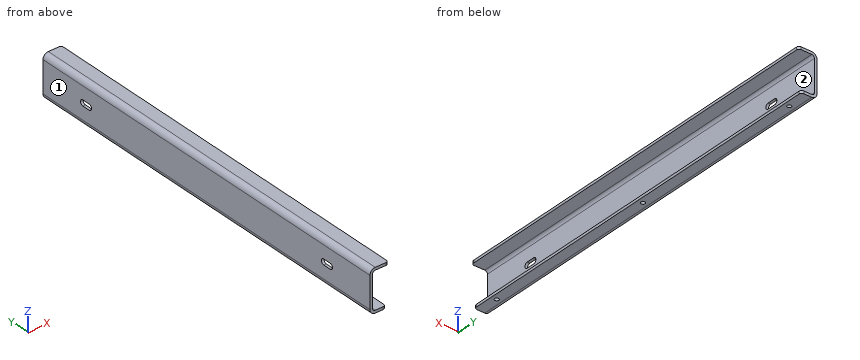
```python
from build123d import *

# Parameters (mm, degrees)
BASE_FLANGE1_DEPTH = 482.6
SKETCH6_R          = 2.45745
CUT_EXTRUDE1_DEPTH = 3.175
FILLET1_R          = 3.175
CUT_EXTRUDE3_DEPTH = 3.175


# Sheet-metal steps are written as plain solids
with BuildPart() as part:
    # Sketch1 → Base-Flange1 (new body)
    with BuildSketch(Plane(origin=(0, 0, 0), x_dir=(1, 0, 0), z_dir=(0, 1, 0))):
        with BuildLine():
            Line((0, 0), (-15.875, 0))
            ThreePointArc((-15.875, 0), (-20.365128061, 1.859871939), (-22.225, 6.35))
            Line((-22.225, 6.35), (-22.225, 44.45))
            ThreePointArc((-22.225, 44.45), (-20.365128061, 48.940128061), (-15.875, 50.8))
            Line((-15.875, 50.8), (-3.175, 50.8))
            Line((-3.175, 50.8), (-3.175, 47.625))
            Line((-3.175, 47.625), (-15.875, 47.625))
            ThreePointArc((-15.875, 47.625), (-18.12006403, 46.69506403), (-19.05, 44.45))
            Line((-19.05, 44.45), (-19.05, 6.35))
            ThreePointArc((-19.05, 6.35), (-18.12006403, 4.10493597), (-15.875, 3.175))
            Line((-15.875, 3.175), (0, 3.175))
            Line((0, 3.175), (0, 0))
        make_face()
    extrude(amount=BASE_FLANGE1_DEPTH)

    # Sketch6 → Cut-Extrude1 (cut)
    with BuildSketch(Plane(origin=(0, 0, -50.8), x_dir=(-1, 0, 0), z_dir=(0, 0, -1))):
        with Locations((9.525, 457.2)):
            Circle(SKETCH6_R)
        with Locations((9.525, 25.4)):
            Circle(SKETCH6_R)
        with Locations((9.525, 241.3)):
            Circle(SKETCH6_R)
    extrude(amount=-CUT_EXTRUDE1_DEPTH, mode=Mode.SUBTRACT)

    # Fillet1
    fillet1_edges = [part.edges().sort_by_distance(p)[0] for p in [
        (-3.175, 0, -49.2125),
        (0, 0, -1.5875),
        (-3.175, 482.6, -49.2125),
        (0, 482.6, -1.5875),
    ]]
    fillet(fillet1_edges, radius=FILLET1_R)

    # Sketch8 → Cut-Extrude3 (cut)
    with BuildSketch(Plane.ZY.offset(22.225)):
        with BuildLine():
            Line((-22.0265625, 423.8625), (-22.0265625, 414.3375))
            ThreePointArc((-22.0265625, 414.3375), (-25.4, 410.9640625), (-28.7734375, 414.3375))
            Line((-28.7734375, 414.3375), (-28.7734375, 423.8625))
            ThreePointArc((-28.7734375, 423.8625), (-25.4, 427.2359375), (-22.0265625, 423.8625))
        make_face()
        with BuildLine():
            Line((-28.7734375, 58.7375), (-28.7734375, 68.2625))
            ThreePointArc((-28.7734375, 68.2625), (-25.4, 71.6359375), (-22.0265625, 68.2625))
            Line((-22.0265625, 68.2625), (-22.0265625, 58.7375))
            ThreePointArc((-22.0265625, 58.7375), (-25.4, 55.3640625), (-28.7734375, 58.7375))
        make_face()
    extrude(amount=-CUT_EXTRUDE3_DEPTH, mode=Mode.SUBTRACT)


solid = part.part
```
Source: CAD feature listing. Evaluate the final solid. Frame: model axes, mm. Face numbers are marked on the shaded views. Coordinates: 2 decimals unless noted, no trailing zeros. Loops run counter-clockwise (first coordinate to the right, second up) from the corner with the lowest first, then second, coordinate; pieces in that order, holes last. Notation, with made-up numbers: M 84.25,-10.5 L 133.25,-10.5 A25 ccw 133.25,16.5 Z; hole C 56.25,6.5 d3. An arc over 180 degrees is marked long. Put each result on its own line as item: value. Start each with the question number.
1) Cut plane A-A on y = 264. Return the cut outline in (x, z) (3 decimals).
2) Ray query, L1, parallel to X at y = 241, z = -50 (3 decimals); L2, parallel to Z at x = -14.5, y = 51 (3 decimals); L3, parallel to X at y = 25, z = -50 (3 decimals). Return the intervals inside material, ascending. Write a range as from..to.
3) Cut plane B-B on z = -33.5. Return the cut outline in (x, y) (3 decimals).
4) Pull-direction query (Z, two-part tool) for the marked faces 1 and 2; classes: pulls with the +Z half, pulls with the -Z half, needs draft (parallel to the pull), parting line crosses it, or undercut.
5) Contact query for flat-ended pins moving along their axis: pin 1 Ø4.5 at (x, y) = (-9.525, 241.3) entering from -Z (3 decimals); pin 2 Ø6 at (y, z) = (268.5, -34.5) entering from +X; pin 3 Ø1.6 at (x, y) = (-21.5, 417) entering from -Z; pin 4 Ø6 at (x, z) = (-4.5, -43.5) entering from -Y. Output: stop coordinate, or through.
The answers:
1. outline: M -22.225,-44.45 A6.35 ccw -15.875,-50.8 L -3.175,-50.8 L -3.175,-47.625 L -15.875,-47.625 A3.175 cw -19.05,-44.45 L -19.05,-6.35 A3.175 cw -15.875,-3.175 L 0,-3.175 L 0,0 L -15.875,0 A6.35 ccw -22.225,-6.35 Z
2. L1: x = -18.96..-11.964, -7.086..-3.175
2. L2: z = -50.8..-47.625, -3.175..0
2. L3: x = -18.96..-11.95, -7.1..-3.175
3. outline: M -22.225,0 L -19.05,0 L -19.05,482.6 L -22.225,482.6 Z
4. face 1: needs draft
4. face 2: undercut
5. pin 1: stops at z = -3.175
5. pin 2: stops at x = -19.05
5. pin 3: stops at z = -48.58
5. pin 4: passes through
